Part model, mm, in its own coordinate system. Coordinates: 2 decimals unless noted, no trailing zeros. Loops run counter-clockwise (first coordinate to the right, second up) from the corner with the lowest first, then second, coordinate; pieces in that order, holes last. Notation, with made-up numbers: (12.25, 34.25) -> (58.25, 34.25) arc R28 ccw to (58.25, 56.25) -> close; hole circle Ø7 at (12.5, 8.5). An arc over 180 degrees is marked (long way). One line per question, with ' | ' between items. Start each with the question number.
1) Probe L1, parallel to Z at x = 2.5, y = 0.4; L2, parallel to Y at x = 13, z = 18.5; L3, parallel to X at y = 0.5, z = -9 (3 decimals). List the from-to ranges inside material, lowest first. Write a range as from..to.
2) Cut at C-C (z = 16). List the corners of the cut face in (x, y) (3 decimals), plus the area to 3 significant figures.
3) Cut at B-B (z = -7). List the corners of the cut face in (x, y) (3 decimals), plus the area to 3 significant figures.
4) Drop a flat-ended pin along its axis: pin 1 (4 mm diameter, centred on x = -33.615, z = -14.516, fed in from -Y). Give the stop position or say it passes through.
5) Cut at D-D (x = -30). List the corners of the cut face in (y, z), plus the area to 3 significant figures.
6) Cut at A-A (x = -12). List the corners of the cut face in (y, z).
Autodesk Fusion 360 part; units mm, degrees
sketch "Esquisse1" plane through (0, 0, 0) normal (0, 1, 0) x (1, 0, 0)
  line L0 (36.115, 26.289) -> (-36.115, 26.289)
  line L1 (-36.115, 26.289) -> (-36.115, -26.289)
  line L2 (-36.115, -26.289) -> (36.115, -26.289)
  line L3 (36.115, -26.289) -> (36.115, 26.289)
  line L4 (36.115, 26.289) -> (-36.115, -26.289) construction
  line L5 (-36.115, 26.289) -> (36.115, -26.289) construction
  line L6 (36.115, 0) -> (31.115, 0) construction
  circle A0 centre (33.615, 0) radius 1.5
  line L7 (33.615, 0) -> (33.615, -14.516) construction
  circle A1 centre (33.615, -14.516) radius 1.5
  circle A2 centre (33.615, 14.516) radius 1.5
  line L8 (0, 0) -> (0, -26.289) construction
  circle A3 centre (-33.615, -14.516) radius 1.5
  circle A4 centre (-33.615, 0) radius 1.5
  circle A5 centre (-33.615, 14.516) radius 1.5
  line L9 (25, 15) -> (-25, 15)
  line L10 (-25, 15) -> (-25, -15)
  line L11 (-25, -15) -> (25, -15)
  line L12 (25, -15) -> (25, 15)
  line L13 (25, 15) -> (-25, -15) construction
  line L14 (-25, 15) -> (25, -15) construction
  dimension "d1" = 72.23
  dimension "d2" = 52.578
  dimension "d5" = 5
  dimension "d6" = 3
  dimension "d7" = 14.516
  dimension "d8" = 3
  dimension "d9" = 50
  dimension "d10" = 30
extrude "Extrusion1" add sketch "Esquisse1" along normal blind 1 contours L0 L1 L2 L3 | A0 | A4
sketch "Sketch2" plane through (0, 1, 0) normal (0, 1, 0) x (-1, 0, 0)
  line L0 (-25, -15) -> (-25, 15)
  line L1 (-25, 15) -> (25, 15)
  line L2 (25, 15) -> (25, -15)
  line L3 (25, -15) -> (-25, -15)
  circle A0 centre (33.615, 14.516) radius 1.5
  circle A1 centre (33.615, -14.516) radius 1.5
  circle A2 centre (-33.615, -14.516) radius 1.5
  circle A3 centre (-33.615, 14.516) radius 1.5
  line L4 (-36.115, 26.289) -> (-36.115, -26.289)
  line L5 (-36.115, -26.289) -> (36.115, -26.289)
  line L6 (36.115, -26.289) -> (36.115, 26.289)
  line L7 (36.115, 26.289) -> (-36.115, 26.289)
  circle A4 centre (-33.615, 14.516) radius 2.5
  circle A5 centre (33.615, 14.516) radius 2.5
  circle A6 centre (33.615, -14.516) radius 2.5
  circle A7 centre (-33.615, -14.516) radius 2.5
  dimension "d13" = 5
  dimension "d14" = 5
  dimension "d15" = 5
  dimension "d16" = 5
extrude "Extrude3" cut sketch "Sketch2" against normal blind 1 contours A4 | A7 | A6 | A5
extrude "Extrude2" add sketch "Esquisse1" against normal blind 5 contours A0 | A4
extrude "Extrude4" add 1 faces at (-12.0383, 0.6667, 26.289) along direction (0, 0, 1) blind 16.5
extrude "Extrude5" add 1 faces at (12.0383, 0.6667, -26.289) along direction (0, 0, -1) blind 16.5
equation "d2 = 39.032 mm + ( 6.773 * 2 ) * 1 mm"
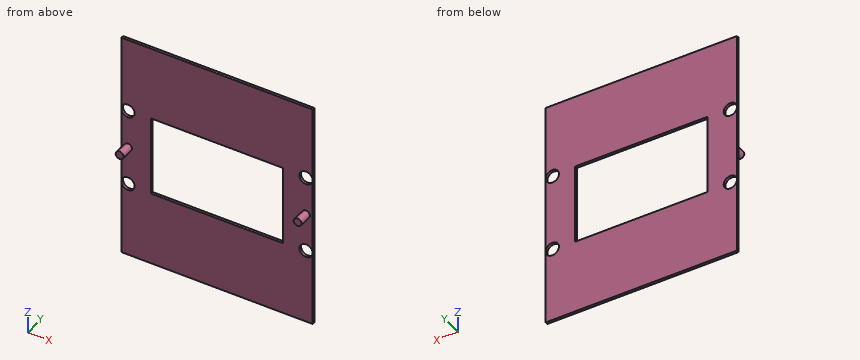
Reported:
1) L1: z = -42.79..-15, 15..42.79 | L2: y = 0..1 | L3: x = -36.115..-25, 25..36.115
2) outline: (-36.115, 0) -> (-35.627, 0) -> (-35.627, 1) -> (-36.115, 1) -> close; (-31.603, 0) -> (31.603, 0) -> (31.603, 1) -> (-31.603, 1) -> close; (35.627, 0) -> (36.115, 0) -> (36.115, 1) -> (35.627, 1) -> close | area: 64.2 mm²
3) outline: (-36.115, 0) -> (-25, 0) -> (-25, 1) -> (-36.115, 1) -> close; (25, 0) -> (36.115, 0) -> (36.115, 1) -> (25, 1) -> close | area: 22.2 mm²
4) pin 1: passes through
5) outline: (0, -42.79) -> (1, -42.79) -> (1, 42.79) -> (0, 42.79) -> close | area: 85.6 mm²
6) outline: (0, -42.79) -> (1, -42.79) -> (1, -15) -> (0, -15) -> close; (0, 15) -> (1, 15) -> (1, 42.79) -> (0, 42.79) -> close
